```python
from build123d import *

# Parameters (mm, degrees)
ESQUISSE1_R                                        = 12
BOSS_EXTRU_1_DEPTH                                 = 3.91
ESQUISSE6_R                                        = 4
ENL_V_MAT_EXTRU_2_DEPTH                            = 1.91
ESQUISSE7_R                                        = 4.95
BOSS_EXTRU_2_DEPTH                                 = 20
CHAMBRAGE_POUR_VIS_T_TE_RONDE_BOMB_E_M_D           = 2.4
CHAMBRAGE_POUR_VIS_T_TE_RONDE_BOMB_E_M_CBORE_D     = 5
CHAMBRAGE_POUR_VIS_T_TE_RONDE_BOMB_E_M_CBORE_DEPTH = 1.6
R_P_TITION_CIRCULAIRE2_COUNT                       = 4


with BuildPart() as part:
    # Esquisse1 → Boss.-Extru.1 (new body)
    with BuildSketch(Plane.XY):
        Circle(ESQUISSE1_R)
    extrude(amount=BOSS_EXTRU_1_DEPTH)

    # Esquisse6 → Enlèv. mat.-Extru.2 (cut)
    with BuildSketch(Plane(origin=(0, 0, 0), x_dir=(-1, 0, 0), z_dir=(0, 0, -1))):
        Circle(ESQUISSE6_R)
    extrude(amount=-ENL_V_MAT_EXTRU_2_DEPTH, mode=Mode.SUBTRACT)

    # Esquisse7 → Boss.-Extru.2 (add)
    with BuildSketch(Plane.XY.offset(3.91)):
        Circle(ESQUISSE7_R)
        with BuildLine():
            Line((1.913896549, 2.445), (-1.913896549, 2.445))
            ThreePointArc((-1.913896549, 2.445), (0, -3.105), (1.913896549, 2.445))
        make_face(mode=Mode.SUBTRACT)
    extrude(amount=BOSS_EXTRU_2_DEPTH)

    # Chambrage pour vis à tête ronde bombée M21 (through all)
    with Locations(Plane.XY.offset(3.91)):
        with Locations((0, 8)):
            chambrage_pour_vis_t_te_ronde_bomb_e_m = CounterBoreHole(CHAMBRAGE_POUR_VIS_T_TE_RONDE_BOMB_E_M_D / 2, CHAMBRAGE_POUR_VIS_T_TE_RONDE_BOMB_E_M_CBORE_D / 2, CHAMBRAGE_POUR_VIS_T_TE_RONDE_BOMB_E_M_CBORE_DEPTH)

    # Répétition circulaire2: Chambrage pour vis à tête ronde bombée M21 ×4 about axis
    r_p_tition_circulaire2_axis = Axis((0, 0, 0), (0, 0, 1))
    for i in range(1, R_P_TITION_CIRCULAIRE2_COUNT):
        add(chambrage_pour_vis_t_te_ronde_bomb_e_m.rotate(r_p_tition_circulaire2_axis, i * 360 / R_P_TITION_CIRCULAIRE2_COUNT), mode=Mode.SUBTRACT)


solid = part.part
```
The model under review builds one solid part; all positions refer to its coordinate system, in mm. A direction names the side the tool comes from. Coordinates: 2 decimals unless noted, no trailing zeros. Write each loop counter-clockwise with the first axis right and the second up, starting at its lowest first coordinate (ties: lowest second). Pieces come first, ordered by that corner, then holes. Notation, with made-up numbers: (48.5, 68.5) - (97.5, 68.5) arc R13 ccw to (97.5, 77.5) - close; hole circle Ø2 at (-27.75, 20.25). An arc over 180 degrees is marked (long way). Answer in a Markdown table with one row per item. Add a question column.
Q1. Clearance check with flat-ended pins moving along their axes: pin 1 (4 mm diameter, centred on y = -1, z = 19, fed in from -X); pin 2 (1.5 mm diameter, centred on y = -6.5, z = 19.5, fed in from +X); pin 3 (4 mm diameter, centred on x = 0.5, y = 8.5, fed in from +Z); pin 4 (4 mm diameter, centred on x = -8, y = 0, fed in from +Z). State where each tip first meets the part, or that it passes through.
Q2. Consider section D-D on z = 17.75. Give the boundary of the cut face in (x, y) (3 decimals).
Q3. Consider section C-C on x = 8. Give the boundary of the cut face in (y, z), then the cut area to 3 significant figures.
Q4. For faces 1 (the face through (0, 0, 1.91)), 2 (the face through (0.65, -9.01, 1.14)), 3 (the face through (-0.54, 5.56, 3.12)), list the 3-axis set-ups (+Z, -Z, +X, -X, +Y, -Y) from which the entire face can be reached by the end or side of a thin tool; tool diameter is ignored.
Q5. To check wall thickness, follow line 1 along Y through (x, z) = (0, 1.3); line 2 along Y through (x, z) = (0, 3.2); line 3 along Z through (x, y) = (-7.5, 2.5). State the ranges of each line that lie inside material, in increasing order. Write a range as from..to.
Q6. Consider section A-A on x = 0. Give the number of separate pieces and of enclosed holes in the cut face, then the cut area to 3 significant figures.
Q7. Draft analysis for pull direction Y (two halves, no side actions). For faces 4 (the face through (-7, -1, 2.31)), 5 (the face through (-11.99, 0.53, 1.93)), 6 (the face through (3.2, -1, 23.91)), state which applies: +Y half, -Y half, draft (parallel to the pull), parting line (faces both ways), or undercut.
Answers below:
| question | item | result |
|---|---|---|
| 1 | pin 1 | x = -4.95 |
| 1 | pin 2 | through |
| 1 | pin 3 | z = 3.91 |
| 1 | pin 4 | z = 2.31 |
| 2 | outline | circle Ø9.9 at (0, 0); hole (-1.914, 2.445) arc R3.105 ccw (long way) to (1.914, 2.445) - close |
| 3 | outline | (-8.94, 0) - (-1.2, 0) - (-1.2, 2.31) - (-2.5, 2.31) - (-2.5, 3.91) - (-8.94, 3.91) - close; (1.2, 0) - (8.94, 0) - (8.94, 3.91) - (2.5, 3.91) - (2.5, 2.31) - (1.2, 2.31) - close |
| 3 | area | 56.4 mm² |
| 4 | face 1 | -Z |
| 4 | face 2 | +Z, -Z |
| 4 | face 3 | +Z |
| 5 | line 1 | -12..-9.2, -6.8..-4, 4..6.8, 9.2..12 |
| 5 | line 2 | -12..-10.5, -5.5..5.5, 10.5..12 |
| 5 | line 3 | 0..3.91 |
| 6 | separate pieces | 3 |
| 6 | enclosed holes | 0 |
| 6 | area | 138 mm² |
| 7 | face 4 | undercut |
| 7 | face 5 | parting line |
| 7 | face 6 | draft |
